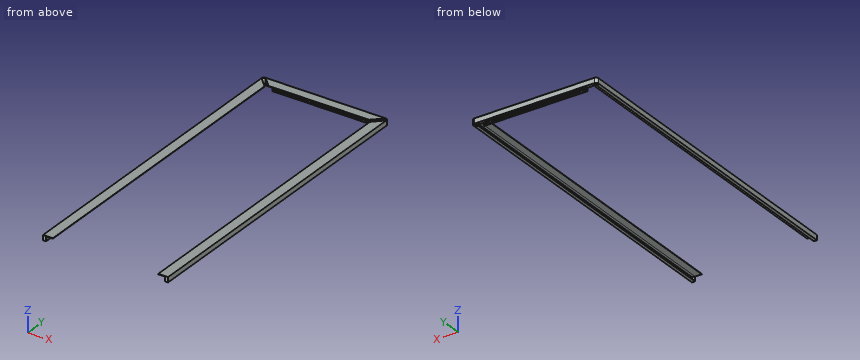
```python
from build123d import *

# Parameters (mm, degrees)
SKETCH1_W           = 647.7
SKETCH1_H           = 1663.7
BOSS_EXTRUDE1_DEPTH = 26.162
SKETCH2_W           = 546.1
SKETCH2_H           = 1612.9
CUT_EXTRUDE1_DEPTH  = 26.162
CUT_EXTRUDE2_DEPTH  = 26.162
CUT_EXTRUDE3_DEPTH  = 24.13
FILLET1_R           = 12.7
SHELL4_START        = 1.778
SHELL4_DEPTH        = 22.606
SKETCH5_W           = 533.4
SKETCH5_H           = 2.286
BOSS_EXTRUDE3_DEPTH = 16.764
SKETCH7_R           = 3.81
CUT_EXTRUDE5_DEPTH  = 16.764


# Read off the part's stored shape, not the designer's step: Shell4
with BuildPart() as part:
    # Sketch1 → Boss-Extrude1 (new body)
    with BuildSketch(Plane.XY):
        Rectangle(SKETCH1_W, SKETCH1_H)
    extrude(amount=BOSS_EXTRUDE1_DEPTH)

    # Sketch2 → Cut-Extrude1 (cut)
    with BuildSketch(Plane.XY.offset(26.162)):
        with Locations((0, -25.4)):
            Rectangle(SKETCH2_W, SKETCH2_H)
    extrude(amount=-CUT_EXTRUDE1_DEPTH, mode=Mode.SUBTRACT)

    # Sketch3 → Cut-Extrude2 (cut)
    with BuildSketch(Plane.XY.offset(26.162)):
        with BuildLine():
            Line((-317.951280605, 813.251280605), (-273.05, 768.35))
            Line((-273.05, 768.35), (-273.05, 781.05))
            Line((-273.05, 781.05), (-260.35, 781.05))
            Line((-260.35, 781.05), (-305.950453026, 825.241047594))
            ThreePointArc((-305.950453026, 825.241047594), (-317.94851482, 825.249344949), (-317.951280605, 813.251280605))
        make_face()
        with BuildLine():
            Line((305.950453026, 825.241047594), (260.35, 781.05))
            Line((260.35, 781.05), (273.05, 781.05))
            Line((273.05, 781.05), (273.05, 768.35))
            Line((273.05, 768.35), (317.951280605, 813.251280605))
            ThreePointArc((317.951280605, 813.251280605), (317.94851482, 825.249344949), (305.950453026, 825.241047594))
        make_face()
    extrude(amount=-CUT_EXTRUDE2_DEPTH, mode=Mode.SUBTRACT)

    # Sketch4 → Cut-Extrude3 (cut)
    with BuildSketch(Plane(origin=(0, 0, 0), x_dir=(-1, 0, 0), z_dir=(0, 0, -1))):
        Polygon((-307.8988, 768.35), (-307.8988, 803.1988), (-273.05, 768.35), (-273.05, -831.85), (-307.8988, -831.85), align=None)
        Polygon((-260.35, 781.05), (-295.735951532, 815.342252918), (295.735951532, 815.342252918), (260.35, 781.05), align=None)
        Polygon((307.8988, 803.1988), (273.05, 768.35), (273.05, -831.85), (307.8988, -831.85), (307.8988, 768.35), align=None)
    extrude(amount=-CUT_EXTRUDE3_DEPTH, mode=Mode.SUBTRACT)

    # Fillet1
    fillet1_edges = [part.edges().sort_by_distance(p)[0] for p in [
        (-323.85, 831.85, 13.081),
        (323.85, 831.85, 13.081),
    ]]
    fillet(fillet1_edges, radius=FILLET1_R)

    # Shell4 outline → Shell4 (cut)
    with BuildSketch(Plane.XY.offset(SHELL4_START)):
        with BuildLine():
            Line((307.8988, 803.1988), (307.8988, -830.072))
            Line((307.8988, -830.072), (322.072, -830.072))
            Line((322.072, -830.072), (322.072, 817.550302353))
            ThreePointArc((322.072, 817.550302353), (321.07369087, 814.548798877), (319.208516462, 811.994044748))
            Line((319.208516462, 811.994044748), (317.951280605, 813.251280605))
            Line((317.951280605, 813.251280605), (307.8988, 803.1988))
        make_face()
        with BuildLine():
            Line((-322.072, -830.072), (-307.8988, -830.072))
            Line((-307.8988, -830.072), (-307.8988, 803.1988))
            Line((-307.8988, 803.1988), (-317.951280605, 813.251280605))
            Line((-317.951280605, 813.251280605), (-319.208516462, 811.994044748))
            ThreePointArc((-319.208516462, 811.994044748), (-321.07369087, 814.548798877), (-322.072, 817.550302353))
            Line((-322.072, 817.550302353), (-322.072, -830.072))
        make_face()
        with BuildLine():
            ThreePointArc((301.905011396, 821.320641288), (309.142763578, 829.116339567), (319.402097182, 826.304926702))
            ThreePointArc((319.402097182, 826.304926702), (315.685635268, 829.085698099), (311.15, 830.072))
            Line((311.15, 830.072), (-311.15, 830.072))
            ThreePointArc((-311.15, 830.072), (-315.685635267, 829.085698099), (-319.402097181, 826.304926702))
            ThreePointArc((-319.402097181, 826.304926702), (-309.142763577, 829.116339567), (-301.905011396, 821.320641288))
            Line((-301.905011396, 821.320641288), (-295.735951532, 815.342252918))
            Line((-295.735951532, 815.342252918), (295.735951532, 815.342252918))
            Line((295.735951532, 815.342252918), (301.905011396, 821.320641288))
        make_face()
    extrude(amount=SHELL4_DEPTH, mode=Mode.SUBTRACT)

    # Sketch5 → Boss-Extrude3 (add)
    with BuildSketch(Plane(origin=(0, 0, 0), x_dir=(-1, 0, 0), z_dir=(0, 0, -1))):
        with Locations((-3.635951532, 816.485252918)):
            Rectangle(SKETCH5_W, SKETCH5_H)
    extrude(amount=BOSS_EXTRUDE3_DEPTH)

    # Sketch7 → Cut-Extrude5 (cut)
    with BuildSketch(Plane(origin=(0, 817.628252918, 0), x_dir=(1, 0, 0), z_dir=(0, 1, 0))):
        with Locations(Location((-256.714048468, 8.382, 0), (0, 0, 270))):
            Circle(SKETCH7_R)
        with Locations(Location((-241.982048468, 8.382, 0), (0, 0, 270))):
            Circle(SKETCH7_R)
        with Locations(Location((-227.250048468, 8.382, 0), (0, 0, 270))):
            Circle(SKETCH7_R)
        with Locations(Location((-212.518048468, 8.382, 0), (0, 0, 270))):
            Circle(SKETCH7_R)
        with Locations(Location((-197.786048468, 8.382, 0), (0, 0, 270))):
            Circle(SKETCH7_R)
        with Locations(Location((-183.054048468, 8.382, 0), (0, 0, 270))):
            Circle(SKETCH7_R)
        with Locations(Location((-168.322048468, 8.382, 0), (0, 0, 270))):
            Circle(SKETCH7_R)
        with Locations(Location((-153.590048468, 8.382, 0), (0, 0, 270))):
            Circle(SKETCH7_R)
        with Locations(Location((-138.858048468, 8.382, 0), (0, 0, 270))):
            Circle(SKETCH7_R)
        with Locations(Location((-124.126048468, 8.382, 0), (0, 0, 270))):
            Circle(SKETCH7_R)
        with Locations(Location((-109.394048468, 8.382, 0), (0, 0, 270))):
            Circle(SKETCH7_R)
        with Locations(Location((-94.662048468, 8.382, 0), (0, 0, 270))):
            Circle(SKETCH7_R)
        with Locations(Location((-79.930048468, 8.382, 0), (0, 0, 270))):
            Circle(SKETCH7_R)
        with Locations(Location((-65.198048468, 8.382, 0), (0, 0, 270))):
            Circle(SKETCH7_R)
        with Locations(Location((-50.466048468, 8.382, 0), (0, 0, 270))):
            Circle(SKETCH7_R)
        with Locations(Location((-35.734048468, 8.382, 0), (0, 0, 270))):
            Circle(SKETCH7_R)
        with Locations(Location((-21.002048468, 8.382, 0), (0, 0, 270))):
            Circle(SKETCH7_R)
        with Locations(Location((-6.270048468, 8.382, 0), (0, 0, 270))):
            Circle(SKETCH7_R)
        with Locations(Location((8.461951532, 8.382, 0), (0, 0, 270))):
            Circle(SKETCH7_R)
        with Locations(Location((23.193951532, 8.382, 0), (0, 0, 270))):
            Circle(SKETCH7_R)
        with Locations(Location((37.925951532, 8.382, 0), (0, 0, 270))):
            Circle(SKETCH7_R)
        with Locations(Location((52.657951532, 8.382, 0), (0, 0, 270))):
            Circle(SKETCH7_R)
        with Locations(Location((67.389951532, 8.382, 0), (0, 0, 270))):
            Circle(SKETCH7_R)
        with Locations(Location((82.121951532, 8.382, 0), (0, 0, 270))):
            Circle(SKETCH7_R)
        with Locations(Location((96.853951532, 8.382, 0), (0, 0, 270))):
            Circle(SKETCH7_R)
        with Locations(Location((111.585951532, 8.382, 0), (0, 0, 270))):
            Circle(SKETCH7_R)
        with Locations(Location((126.317951532, 8.382, 0), (0, 0, 270))):
            Circle(SKETCH7_R)
        with Locations(Location((141.049951532, 8.382, 0), (0, 0, 270))):
            Circle(SKETCH7_R)
        with Locations(Location((155.781951532, 8.382, 0), (0, 0, 270))):
            Circle(SKETCH7_R)
        with Locations(Location((170.513951532, 8.382, 0), (0, 0, 270))):
            Circle(SKETCH7_R)
        with Locations(Location((185.245951532, 8.382, 0), (0, 0, 270))):
            Circle(SKETCH7_R)
        with Locations(Location((199.977951532, 8.382, 0), (0, 0, 270))):
            Circle(SKETCH7_R)
        with Locations(Location((214.709951532, 8.382, 0), (0, 0, 270))):
            Circle(SKETCH7_R)
        with Locations(Location((229.441951532, 8.382, 0), (0, 0, 270))):
            Circle(SKETCH7_R)
        with Locations(Location((244.173951532, 8.382, 0), (0, 0, 270))):
            Circle(SKETCH7_R)
        with Locations(Location((258.905951532, 8.382, 0), (0, 0, 270))):
            Circle(SKETCH7_R)
    extrude(amount=-CUT_EXTRUDE5_DEPTH, mode=Mode.SUBTRACT)


solid = part.part
```
Design review of the part built by this model. Coordinates are the model's own, in mm. Coordinates: 2 decimals unless noted, no trailing zeros. Order: outer loops, then holes, each group sorted by start corner. A loop starts at its lowest first (then second) coordinate and runs counter-clockwise, first axis right, second up.
1) Wall thickness on line 1 along X through (y, z) = (489, 21.5); line 2 along Y through (x, z) = (107, 12); line 3 along Y through (x, z) = (-41, 0.5): over which ranges is each line inside the solid? List them lowest first.
2) Take a section at B-B, the plane z = 9. Give the boundary of the cut face in (x, y).
3) Clearance check with flat-ended pins moving along their axes: pin 1 (25 mm diameter, centred on x = -43, z = 10, fed in from -Y); pin 2 (0.6 mm diameter, centred on x = 107, z = 24.5, fed in from -Y); pin 3 (4.5 mm diameter, centred on x = 315.5, y = -336, fed in from -Z). State where each tip first meets the part, or that it passes through.
4) Take a section at A-A, the plane y = 513.5. Give the boundary of the cut face in (x, z).
Returned:
1. line 1: x = -323.85 to -322.07, 322.07 to 323.85
1. line 2: y = 830.07 to 831.85
1. line 3: y = 815.34 to 831.85
2. outline: (-323.85, -831.85) - (-307.9, -831.85) - (-307.9, -830.07) - (-322.07, -830.07) - (-322.07, 817.55) arc R10.26 ccw to (-319.21, 811.99) - (-317.95, 813.25) arc R8.48 cw to (-305.95, 825.24) - (-301.91, 821.32) arc R10.26 ccw to (-319.4, 826.3) arc R10.92 cw to (-311.15, 830.07) - (311.15, 830.07) arc R10.92 cw to (319.4, 826.3) arc R10.26 ccw to (301.91, 821.32) - (305.95, 825.24) arc R8.48 cw to (317.95, 813.25) - (319.21, 811.99) arc R10.26 ccw to (322.07, 817.55) - (322.07, -830.07) - (307.9, -830.07) - (307.9, -831.85) - (323.85, -831.85) - (323.85, 819.15) arc R12.7 ccw to (311.15, 831.85) - (-311.15, 831.85) arc R12.7 ccw to (-323.85, 819.15) - close
3. pin 1: stops at y = 815.34
3. pin 2: stops at y = 781.05
3. pin 3: stops at z = 0
4. outline: (-323.85, 0) - (-307.9, 0) - (-307.9, 1.78) - (-322.07, 1.78) - (-322.07, 24.38) - (-307.9, 24.38) - (-307.9, 24.13) - (-273.05, 24.13) - (-273.05, 26.16) - (-323.85, 26.16) - close; (273.05, 24.13) - (307.9, 24.13) - (307.9, 24.38) - (322.07, 24.38) - (322.07, 1.78) - (307.9, 1.78) - (307.9, 0) - (323.85, 0) - (323.85, 26.16) - (273.05, 26.16) - close
